Source: three-view drawing plus pictorial views. Frame: mm from the lowest corner of the part. A direction names the side the tool comes from. Round coordinates to 2 decimals unless told otherwise and drop trailing zeros. Loops run counter-clockwise (first coordinate to the right, second up) from the corner with the lowest first, then second, coordinate; pieces in that order, holes last. Notation, with made-up numbers: (-15, -11) -> (-5, -11) arc R17 cw to (-5, -2) -> close; hole circle Ø10 at (-11.5, 54.5). An arc over 180 degrees is marked (long way). Answer as a JSON object with one key per item and string values. Group by question number.
Item 1: Section query A-A on x = 31. Return loops of the section in (y, z).
Item 2: Set-up query: the marked faces 1 and 2. Return all of +Z, -Z, +X, -X, +Y, -Y with unobstructed straight access to the full face (end or side cutting, diameter ignored); none if empty.
Item 3: Section query B-B on z = 15. Return loops of the section in (x, y) (1 decimal).
Item 4: Pin query (flat end, axial travel): pin 1 (3 mm diameter, centred on x = 33, z = 53.5, fed in from -Y); pin 2 (12.5 mm diameter, centred on x = 30, z = 11.5, fed in from +Y); pin 3 (5 mm diameter, centred on x = 55, y = 97.5, fed in from -Z). Return the tip coordinate at first contact, or that it passes through.
Item 5: Material intervals for line 1 (Y direction, x = 48, z = 48.5); line 2 (X direction, y = 12.5, z = 10.5) (1 decimal); line 3 (Y direction, x = 48, z = 18.5), sorted ascending. Write a range as [from, to].
Item 6: Section query C-C on y = 111. Return loops of the section in (x, z), and give its area (3 significant figures).
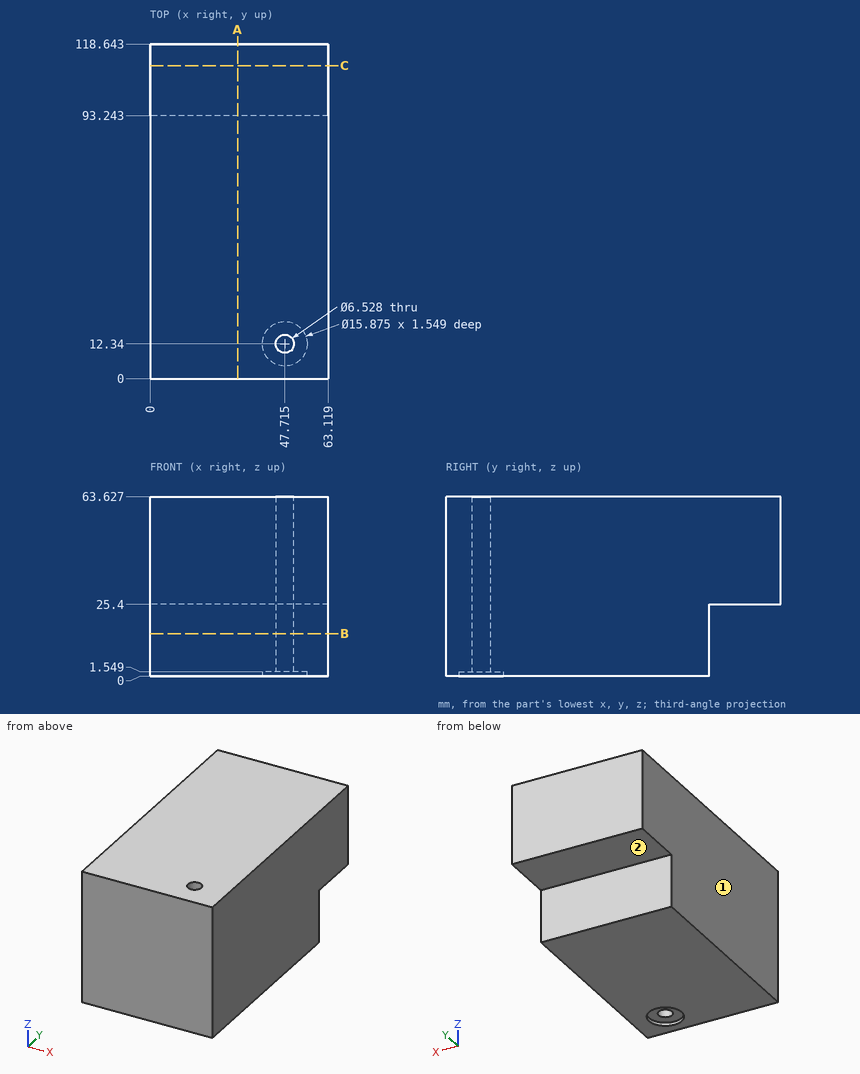
Solved:
{
 "1": {"outline": "(0, 0) -> (93.24, 0) -> (93.24, 25.4) -> (118.64, 25.4) -> (118.64, 63.63) -> (0, 63.63) -> close"},
 "2": {"face 1": "+Z, -Z, -X, +Y, -Y", "face 2": "-Z, +X, -X, +Y"},
 "3": {"outline": "(0, 0) -> (63.1, 0) -> (63.1, 93.2) -> (0, 93.2) -> close; hole circle Ø6.5 at (47.7, 12.3)"},
 "4": {"pin 1": "y = 0", "pin 2": "y = 93.24", "pin 3": "z = 25.4"},
 "5": {"line 1": "[0, 9.09], [15.59, 118.64]", "line 2": "[0, 44.5], [51, 63.1]", "line 3": "[0, 9.09], [15.59, 93.24]"},
 "6": {"outline": "(0, 25.4) -> (63.12, 25.4) -> (63.12, 63.63) -> (0, 63.63) -> close", "area": "2,410 mm²"}
}
